Autodesk Inventor part; units mm, degrees
ref_plane "YZ Plane" through (0, 0, 0) normal (1, 0, 0) x (0, 1, 0)
ref_plane "XZ Plane" through (0, 0, 0) normal (0, 1, 0) x (-1, 0, 0)
ref_plane "XY Plane" through (0, 0, 0) normal (0, 0, 1) x (1, 0, 0)
sketch "Sketch1" plane through (0, 0, 0) normal (0, 1, 0) x (-1, 0, 0)
  line L0 (0, 0) -> (9.652, 0)
  line L1 (9.652, 0) -> (9.652, -38.1)
  line L2 (9.652, -38.1) -> (0, -38.1)
  line L3 (0, -38.1) -> (0, 0)
  dimension "d0" = 9.652
  dimension "d1" = 38.1
extrude "Extrusion1" add sketch "Sketch1" along normal blind 76.2
sketch "Sketch2" plane through (0, 0, 0) normal (1, 0, 0) x (0, 0, -1)
  line L0 (38.1, 0) -> (38.1, 76.2)
  line L1 (0, 76.2) -> (38.1, 76.2)
  line L2 (0, 0) -> (0, 76.2)
  point P0 (6.35, 69.85)
  point P1 (31.75, 69.85)
  dimension "d4" = 6.35
  dimension "d5" = 6.35
  dimension "d6" = 6.35
  dimension "d7" = 6.35
hole "Hole1" at (0, 69.85, -6.35) at (0, 69.85, -31.75) direction (-1, 0, 0) diameter 2.7178 depth 25.4 tip angle 118
properties part number "motor stand"
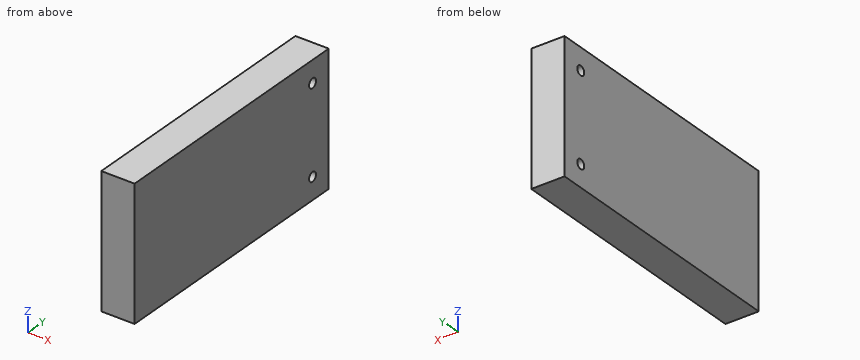
Part model, mm, in its own coordinate system. Round coordinates to 2 decimals unless told otherwise and drop trailing zeros. Loops run counter-clockwise (first coordinate to the right, second up) from the corner with the lowest first, then second, coordinate; pieces in that order, holes last. Notation, with made-up numbers: (30, 3.25) -> (73, 3.25) arc R17 cw to (73, 36.25) -> close; hole circle Ø2 at (70, -36.5). An arc over 180 degrees is marked (long way). Use one line per item in the form item = value. Start each with the question number.
Item 1: Drill centre lines: line 1 along Z through (x, y) = (-5.25, 69.85); line 2 along Y through (x, z) = (-7.5, -31.75). Where is each one in solid material? Low to high.
Item 2: Band-saw the part on A-A (y = 69.85). List the corners of the cut face in (x, z), plus the area to 3 significant figures.
Item 3: Band-saw the part on B-B (z = -6.35). List the corners of the cut face in (x, y).
Data:
q1.line_1 = -38.1 to -33.11, -30.39 to -7.71, -4.99 to 0
q1.line_2 = 0 to 68.49, 71.21 to 76.2
q2.outline = (-9.65, -38.1) -> (0, -38.1) -> (0, -33.11) -> (-9.65, -33.11) -> close; (-9.65, -30.39) -> (0, -30.39) -> (0, -7.71) -> (-9.65, -7.71) -> close; (-9.65, -4.99) -> (0, -4.99) -> (0, 0) -> (-9.65, 0) -> close
q2.area = 315 mm^2
q3.outline = (-9.65, 0) -> (0, 0) -> (0, 68.49) -> (-9.65, 68.49) -> close; (-9.65, 71.21) -> (0, 71.21) -> (0, 76.2) -> (-9.65, 76.2) -> close
